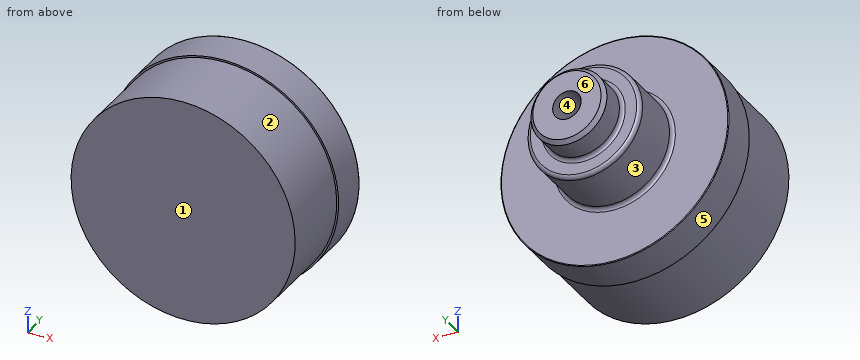
```python
from build123d import *

# Parameters (mm, degrees)
SKETCH1_R                        = 37.465
BOSS_EXTRUDE1_DEPTH              = 25.4
SKETCH2_R                        = 38.1
BOSS_EXTRUDE2_DEPTH              = 12.7
SKETCH3_R                        = 19.05
BOSS_EXTRUDE3_DEPTH              = 19.05
SKETCH4_R                        = 12.7
BOSS_EXTRUDE4_DEPTH              = 10.16
FILLET1_SIZE                     = 1.27
FILLET2_R                        = 1.27
FILLET3_R                        = 0.254
FILLET4_R                        = 1.27
FILLET5_R                        = 1.27
F_3_8_0_375_DIAMETER_HOLE1_D     = 9.525
F_3_8_0_375_DIAMETER_HOLE1_DEPTH = 25.4
F_3_8_0_375_DIAMETER_HOLE1_TIP   = 2.861598698


with BuildPart() as part:
    # Sketch1 → Boss-Extrude1 (new body)
    with BuildSketch(Plane(origin=(0, 0, 0), x_dir=(1, 0, 0), z_dir=(0, 1, 0))):
        with Locations(Location((0, 0, 0), (0, 0, 270))):
            Circle(SKETCH1_R)
    extrude(amount=BOSS_EXTRUDE1_DEPTH)

    # Sketch2 → Boss-Extrude2 (add)
    with BuildSketch(Plane(origin=(0, 25.4, 0), x_dir=(1, 0, 0), z_dir=(0, 1, 0))):
        with Locations(Location((0, 0, 0), (0, 0, 270))):
            Circle(SKETCH2_R)
    extrude(amount=BOSS_EXTRUDE2_DEPTH)

    # Sketch3 → Boss-Extrude3 (add)
    with BuildSketch(Plane(origin=(0, 38.1, 0), x_dir=(1, 0, 0), z_dir=(0, 1, 0))):
        with Locations(Location((0, 0, 0), (0, 0, 90))):
            Circle(SKETCH3_R)
    extrude(amount=BOSS_EXTRUDE3_DEPTH)

    # Sketch4 → Boss-Extrude4 (add)
    with BuildSketch(Plane(origin=(0, 57.15, 0), x_dir=(1, 0, 0), z_dir=(0, 1, 0))):
        with Locations(Location((0, 0, 0), (0, 0, 270))):
            Circle(SKETCH4_R)
    extrude(amount=BOSS_EXTRUDE4_DEPTH)

    # Fillet1
    fillet1_edges = [part.edges().sort_by_distance(p)[0] for p in [
        (0, 67.31, -12.7),
    ]]
    chamfer(fillet1_edges, length=FILLET1_SIZE)

    # Fillet2
    fillet2_edges = [part.edges().sort_by_distance(p)[0] for p in [
        (0, 57.15, 19.05),
    ]]
    fillet(fillet2_edges, radius=FILLET2_R)

    # Fillet3
    fillet3_edges = [part.edges().sort_by_distance(p)[0] for p in [
        (0, 38.1, -38.1),
    ]]
    fillet(fillet3_edges, radius=FILLET3_R)

    # Fillet4
    fillet4_edges = [part.edges().sort_by_distance(p)[0] for p in [
        (0, 38.1, 19.05),
    ]]
    fillet(fillet4_edges, radius=FILLET4_R)

    # Fillet5
    fillet5_edges = [part.edges().sort_by_distance(p)[0] for p in [
        (0, 57.15, -12.7),
    ]]
    fillet(fillet5_edges, radius=FILLET5_R)

    # 3_8 _0.375_ Diameter Hole1
    with Locations(Plane(origin=(0, 67.31, 0), x_dir=(1, 0, 0), z_dir=(0, 1, 0))):
        with Locations((0, 0)):
            Hole(F_3_8_0_375_DIAMETER_HOLE1_D / 2, depth=F_3_8_0_375_DIAMETER_HOLE1_DEPTH)
            with Locations((0, 0, -(F_3_8_0_375_DIAMETER_HOLE1_DEPTH + F_3_8_0_375_DIAMETER_HOLE1_TIP / 2))):  # 118° drill point
                Cone(0, F_3_8_0_375_DIAMETER_HOLE1_D / 2, F_3_8_0_375_DIAMETER_HOLE1_TIP, mode=Mode.SUBTRACT)


solid = part.part
```
Design review of the part built by this model. Coordinates are the model's own, in mm. Face numbers are marked on the shaded views. A direction names the side the tool comes from. Round coordinates to 2 decimals unless told otherwise and drop trailing zeros. Order: outer loops, then holes, each group sorted by start corner. A loop starts at its lowest first (then second) coordinate and runs counter-clockwise, first axis right, second up. Notation, with made-up numbers: (57, 3) - (70, 3) arc R24 ccw to (70, 25) - close; hole circle Ø8 at (32, -18.75). An arc over 180 degrees is marked (long way). Return JSON: item names as keys, results as strings.
Q1. For pin 1 Ø1 at (x, y) = (22, 21.5) entering from -Z; pin 2 Ø1 at (y, z) = (11.5, -3.5) entering from +X; pin 3 Ø8 at (y, z) = (40.5, 26) entering from +X, all flat-tipped, find the tip position at first contact; note any pin that passes through.
Computed values:
{"pin 1": "stops at z = -30.68", "pin 2": "stops at x = 37.34", "pin 3": "stops at x = 30.41"}
Q2. Consider section B-B on y = 13.5. Write out the cut boundary in (x, z) (3 decimals).
Computed values:
{"outline": "circle Ø74.93 at (0, 0)"}
Q3. Consider section C-C on y = 36. Write out the cut boundary in (x, z).
Computed values:
{"outline": "circle Ø76.2 at (0, 0)"}
Q4. Machinability: for the marked faces 1, 2 and 3, which of the approach directions +Z, -Z, +X, -X, +Y, -Y give a long, thin tool a straight path to every point of the face, cutting with its end or side? Answer none if there is none.
Computed values:
{"face 1": "+Z, -Z, +X, -X, -Y", "face 2": "-Y", "face 3": "+Y"}
Q5. The part is to be moulded in two halves that separate along X. For the marked faces 4, 5 and 6, say which applies: pulls with the +X half, pulls with the -X half, needs draft (parallel to the pull), parting line crosses it, or undercut.
Computed values:
{"face 4": "undercut", "face 5": "parting line crosses it", "face 6": "needs draft"}
Q6. Wall thickness on L1, parallel to Z at x = 1, y = 8.5; L2, parallel to Y at x = -21.5, z = 5; L3, parallel to Y at x = 34.5, z = 15: over which ranges is each line inside the solid? List them lowest first. Write a range as [from, to].
Computed values:
{"L1": "z = [-37.45, 37.45]", "L2": "y = [0, 38.1]", "L3": "y = [25.4, 38.1]"}
